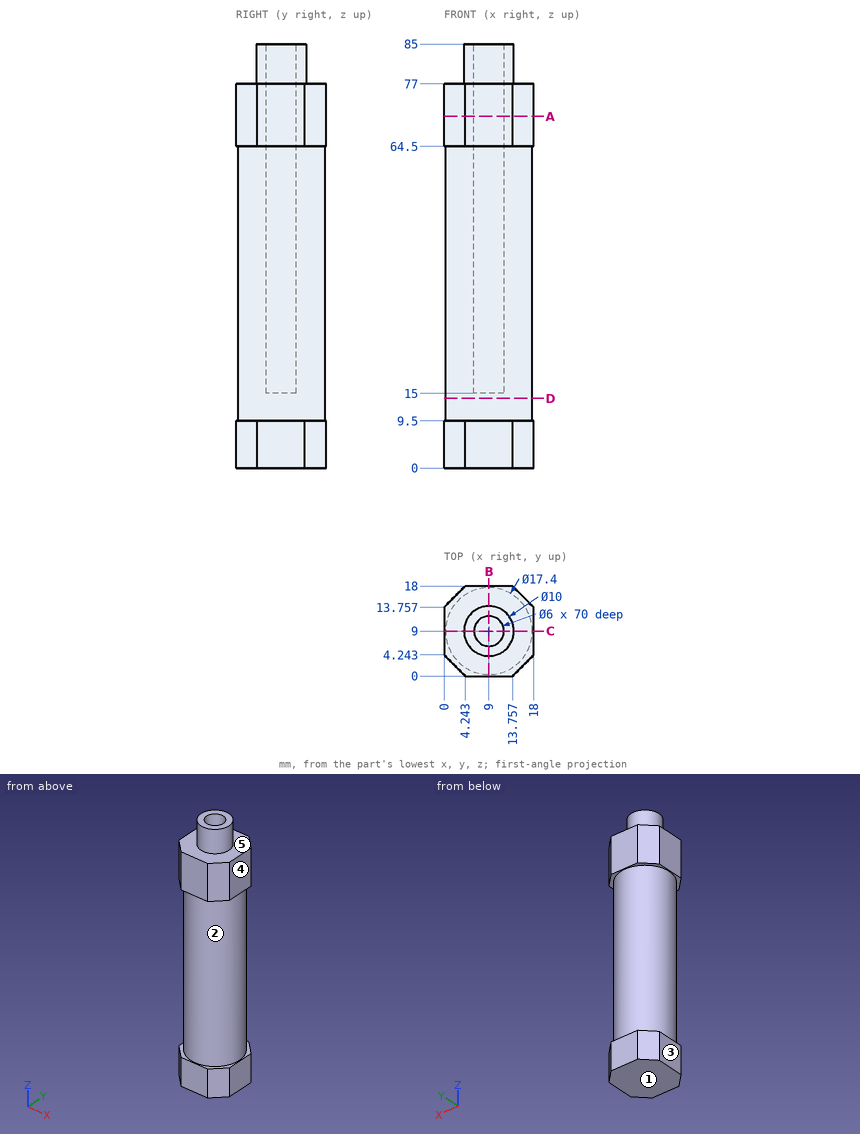
Geometry: see drawing. Coordinates: mm, zero at the bounding-box minimum. A direction names the side the tool comes from. Coordinates: 2 decimals unless noted, no trailing zeros. Write each loop counter-clockwise with the first axis right and the second up, starting at its lowest first coordinate (ties: lowest second). Pieces come first, ordered by that corner, then holes. Notation, with made-up numbers: M 5,-37.5 L 64,-37.5 A28 ccw 64,-10.5 Z; hole C 80.5,-39.5 d7. An arc over 180 degrees is marked long. Answer as a JSON object with one key per item and string values.
1. Draft query along Z for the marked faces 1, 2 and 3. Return one class per face: released by +Z, released by -Z, zero draft, split by the parting line, or undercut.
Evaluation:
{"face 1": "released by -Z", "face 2": "undercut", "face 3": "zero draft"}
2. Cut plane B-B on x = 9. Output: boundary loops of the cut face in (y, z).
Evaluation:
{"outline": "M 0,0 L 18,0 L 18,9.5 L 17.7,9.5 L 17.7,64.5 L 18,64.5 L 18,77 L 14,77 L 14,85 L 12,85 L 12,15 L 6,15 L 6,85 L 4,85 L 4,77 L 0,77 L 0,64.5 L 0.3,64.5 L 0.3,9.5 L 0,9.5 Z"}
3. Cut plane D-D on z = 14. Output: boundary loops of the cut face in (x, y).
Evaluation:
{"outline": "C 9,9 d17.4"}
4. Cut plane A-A on z = 70.5. Output: boundary loops of the cut face in (x, y), plus the area to 3 significant figures.
Evaluation:
{"outline": "M 0,4.24 L 4.24,0 L 13.76,0 L 18,4.24 L 18,13.76 L 13.76,18 L 4.24,18 L 0,13.76 Z; hole C 9,9 d6", "area": "260 mm^2"}
5. Access query for the marked faces 4 and 5. Directions: +Z, -Z, +X, -X, +Y, -Y. A direction counts if a zero-diameter tool reaches every point of the face in a straight line with its end or side. Return the directions, or none.
Evaluation:
{"face 4": "+Z, -Z, +X, +Y, -Y", "face 5": "+Z"}
6. Ray query, L1, parallel to Y at x = 9, z = 35.5; L2, parallel to Z at x = 8.5, y = 2.5; L3, parallel to Z at x = 14.5, y = 1.25. Return the intervals inside material, ascending.
Evaluation:
{"L1": "0.3 to 6, 12 to 17.7", "L2": "0 to 77", "L3": "0 to 9.5, 64.5 to 77"}
7. Contact query for flat-ended pins moving along their axis: P1, Ø3, axis at x = 13.5, y = 3.5, coming from the +Z side; P2, Ø10, axis at y = 15.5, z = 34.5, coming from the -X side; P3, Ø5, axis at y = 9, z = 33, coming from the +X side. Output: stop coordinate, or through.
Evaluation:
{"P1": "z = 77", "P2": "x = 0.43", "P3": "x = 17.7"}
